Check sheet for the modelled part. Datum: model origin and axes. Units: mm. Round coordinates to 2 decimals unless told otherwise and drop trailing zeros. Write each loop counter-clockwise with the first axis right and the second up, starting at its lowest first coordinate (ties: lowest second). Pieces come first, ordered by that corner, then holes. Notation, with made-up numbers: M 89,12 L 95,12 A30 cw 95,49 Z; hole C -1,3 d4. An arc over 180 degrees is marked long. One line per item, written item: value.
Autodesk Inventor part; units mm, degrees
ref_plane "YZ Plane" through (0, 0, 0) normal (1, 0, 0) x (0, 1, 0)
ref_plane "XZ Plane" through (0, 0, 0) normal (0, 1, 0) x (-1, 0, 0)
ref_plane "XY Plane" through (0, 0, 0) normal (0, 0, 1) x (1, 0, 0)
sketch "Esquisse1" plane through (0, 0, 0) normal (0, 1, 0) x (-1, 0, 0)
  arc A0 (15, 0) -> (-15, 0) centre (0, 0) ccw
  line L0 (-15, 0) -> (15, 0) construction
  line L1 (15, 0) -> (15, -25)
  line L2 (15, -25) -> (-15, -25)
  line L3 (-15, -25) -> (-15, 0)
  arc A1 (-15, 0) -> (15, 0) centre (0, 0) ccw construction
  dimension "d0" = 30
  dimension "d1" = 25
extrude "Extrusion1" add sketch "Esquisse1" along normal blind 2
sketch "Esquisse2" plane through (0, 2, 0) normal (0, 1, 0) x (1, 0, 0)
  arc A0 (-15, 0) -> (15, 0) centre (0, 0) ccw
  line L0 (15, 25) -> (-15, 25)
  circle A1 centre (-10, 0) radius 1.25
  circle A2 centre (10, 0) radius 1.25
  line L1 (0, 0) -> (0, 25) construction
  line L2 (0, 0) -> (-15, 0) construction
  dimension "d4" = 2.5
  dimension "d5" = 10
extrude "Extrusion2" cut sketch "Esquisse2" against normal through all
sketch "Esquisse3" plane through (0, 2, 0) normal (0, 1, 0) x (1, 0, 0)
  arc A0 (-15, 0) -> (15, 0) centre (0, 0) ccw
  circle A1 centre (0, 0) radius 5.5
  dimension "d8" = 11
extrude "Extrusion3" cut sketch "Esquisse3" against normal through all
fillet "Congé1" radius 2 2 edges at (-15, 1, -25) (15, 1, -25)
properties part number "encoder_fixation"
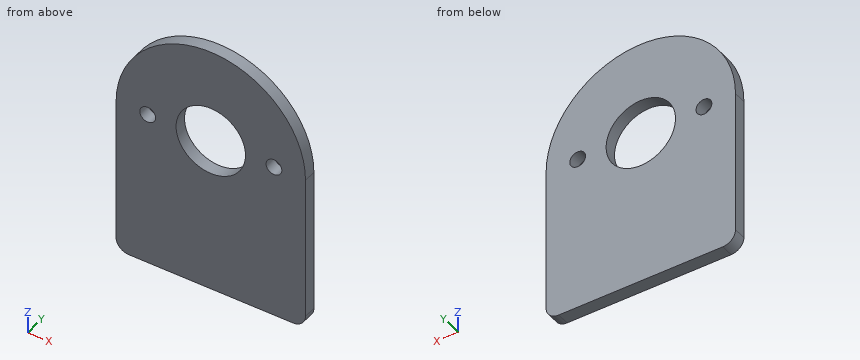
Q1. Sectioned sample at B-B on z = -2. Enter the section's corners in (x, y), and give its area (3 significant figures).
Completed:
outline: M -15,0 L -5.12,0 L -5.12,2 L -15,2 Z; M 5.12,0 L 15,0 L 15,2 L 5.12,2 Z
area: 39.5 mm^2
Q2. Scan lines: line 1 (X direction, y = 1.3, z = 0); line 2 (Z direction, x = 0, y = 0.9); line 3 (Z direction, x = -10, y = 1.6). Record each from-to range of solid material in increasing order. Write a range as [from, to].
Completed:
line 1: [-15, -11.25], [-8.75, -5.5], [5.5, 8.75], [11.25, 15]
line 2: [-25, -5.5], [5.5, 15]
line 3: [-25, -1.25], [1.25, 11.18]
Q3. Sectioned sample at C-C on y = 0.4. Enter the section's corners in (x, z), and give its area (3 significant figures).
Completed:
outline: M -15,-23 A2 ccw -13,-25 L 13,-25 A2 ccw 15,-23 L 15,0 A15 ccw -15,0 Z; hole C -10,0 d2.5; hole C 0,0 d11; hole C 10,0 d2.5
area: 997 mm^2
Q4. Sectioned sample at A-A on x = 0. Enter the section's corners in (y, z), and give its area (3 significant figures).
Completed:
outline: M 0,-25 L 2,-25 L 2,-5.5 L 0,-5.5 Z; M 0,5.5 L 2,5.5 L 2,15 L 0,15 Z
area: 58.0 mm^2
Q5. Depth check by flat-ended pin: P1, Ø10, axis at x = 0, z = 0, coming from the +Y side. Enter the tip coordinate at first touch or a pass-through.
Completed:
P1: through
